Check sheet for the modelled part. Datum: model origin and axes. Units: mm. A direction names the side the tool comes from. Give positions to 0.01 mm unless a question says otherwise; leave off trailing zeros. Order: outer loops, then holes, each group sorted by start corner. A loop starts at its lowest first (then second) coordinate and runs counter-clockwise, first axis right, second up. Notation, with made-up numbers: (-11, 4) - (14, 4) arc R14 cw to (14, 24) - close; hole circle Ø7 at (43.25, 27). An arc over 180 degrees is marked (long way). Answer in a Markdown table with one row per item.
from build123d import *

# Parameters (mm, degrees)
SKETCH5_R           = 3.175
BOSS_EXTRUDE3_DEPTH = 203.2
CHAMFER1_SIZE       = 0.9525
BOSS_EXTRUDE4_DEPTH = 4.365625
SKETCH8_OUTSIDE_W   = 777.858
SKETCH8_OUTSIDE_H   = 779.578
SKETCH8_OUTSIDE_R   = 5.55625
CUT_EXTRUDE3_DEPTH  = 208.739074677
CUT_EXTRUDE3_DRAFT  = -60
CUT_EXTRUDE4_DEPTH  = 0.254
CIRPATTERN1_COUNT   = 6


with BuildPart() as part:
    # Sketch5 → Boss-Extrude3 (new body)
    with BuildSketch(Plane(origin=(103.7828125, 0, 0), x_dir=(0, 0, -1), z_dir=(1, 0, 0))):
        Circle(SKETCH5_R)
    extrude(amount=-BOSS_EXTRUDE3_DEPTH)

    # Chamfer1
    chamfer1_edges = [part.edges().sort_by_distance(p)[0] for p in [
        (103.7828125, 0, 3.175),
    ]]
    chamfer(chamfer1_edges, length=CHAMFER1_SIZE)

    # Sketch11 → Revolve1 (revolve)
    with BuildSketch(Plane.XY):
        Polygon((-99.4171875, 3.175), (-99.4171875, 0), (81.5578125, 0), (78.3828125, 3.175), align=None)
    revolve(axis=Axis((-99.4171875, 0, 0), (1, 0, 0)))

    # Sketch6 → Boss-Extrude4 (add)
    with BuildSketch(Plane.ZY.offset(99.4171875)):
        Polygon((5.55625, 3.207902433), (0, 6.415804866), (-5.55625, 3.207902433), (-5.55625, -3.207902433), (0, -6.415804866), (5.55625, -3.207902433), align=None)
    extrude(amount=BOSS_EXTRUDE4_DEPTH)


with BuildPart() as cut_extrude3_tool:
    # Sketch8 outside → Cut-Extrude3 (with draft: the straight prism first)
    with BuildSketch(Plane.ZY.offset(103.7828125)):
        Rectangle(SKETCH8_OUTSIDE_W, SKETCH8_OUTSIDE_H)
        Circle(SKETCH8_OUTSIDE_R, mode=Mode.SUBTRACT)
    extrude(amount=-CUT_EXTRUDE3_DEPTH)
    # Cut-Extrude3: the draft: its side faces are tilted about the plane it starts from
    cut_extrude3_sides = [cut_extrude3_tool.faces().sort_by_distance(p)[0] for p in [
        (0.586724839, -389.789, 0),
        (0.586724839, 0, 388.929),
        (0.586724839, 389.789, 0),
        (0.586724839, 0, -388.929),
        (0.586724839, 0, -5.55625),
    ]]
    draft(cut_extrude3_sides, Plane.ZY.offset(103.7828125), CUT_EXTRUDE3_DRAFT)


with BuildPart() as part_1:
    add(part.part)

    # Cut-Extrude3: cut by cut_extrude3_tool
    add(cut_extrude3_tool.part, mode=Mode.SUBTRACT)

    # Sketch12 → Cut-Extrude4 (cut)
    with BuildSketch(Plane.ZY.offset(103.7828125)):
        with BuildLine():
            Line((0.1666875, 4.2783125), (0.1666875, 2.3891875))
            ThreePointArc((0.1666875, 2.3891875), (0, 2.2225), (-0.1666875, 2.3891875))
            Line((-0.1666875, 2.3891875), (-0.1666875, 4.2783125))
            ThreePointArc((-0.1666875, 4.2783125), (0, 4.445), (0.1666875, 4.2783125))
        make_face()
    cut_extrude4 = extrude(amount=-CUT_EXTRUDE4_DEPTH, mode=Mode.SUBTRACT)

    # CirPattern1: Cut-Extrude4 ×6 about axis
    cirpattern1_axis = Axis((0, 0, 0), (1, 0, 0))
    for i in range(1, CIRPATTERN1_COUNT):
        add(cut_extrude4.rotate(cirpattern1_axis, i * 360 / CIRPATTERN1_COUNT), mode=Mode.SUBTRACT)


solid = part_1.part
(1) Thickness scan on L1, parallel to X at y = 4.5, z = 2; L2, parallel to Y at x = 92, z = -2.5; L3, parallel to Y at x = -47, z = -2.25. Record the ranges inside material, lowest first.
Geometry says:
| item | result |
|---|---|
| L1 | -103.78 to -99.42 |
| L2 | -1.96 to 1.96 |
| L3 | -2.24 to 2.24 |
(2) Access from +Z, -Z, +X, -X, +Y, -Y to the whole of each face (thin tool, end or side, straight path). Record for faces 1 (the flat face through (-101.569, 4.834, -2.739)), 2 (the cylindrical face through (3.12, -3.1, 0.69)).
Geometry says:
| item | result |
|---|---|
| face 1 | -Z, +X, -X, +Y |
| face 2 | +X |
(3) Cross-section at A-A, the plane x = 76. Record the cut outline in (y, z) (3 decimals).
Geometry says:
| item | result |
|---|---|
| outline | circle Ø6.35 at (0, 0) |
(4) Gauge pin test, flat ends, axial feed: P1, Ø4, axis at x = 79.5, y = -1.5, coming from the -Z side (3 decimals); P2, Ø4, axis at x = 21.5, z = -1.5, coming from the -Y side (3 decimals); P3, Ø2, axis at y = 3.5, z = -2, coming from the +X side. Record the tip position at first contact, or that the pin passes through.
Geometry says:
| item | result |
|---|---|
| P1 | z = -3.175 |
| P2 | y = -3.175 |
| P3 | x = 102.97 |
